The figure shows three views and two pictorial views of one solid part (mm, origin at its lowest corner). Answer the questions. A direction names the side the tool comes from. Coordinates: 2 decimals unless noted, no trailing zeros. Loops run counter-clockwise (first coordinate to the right, second up) from the corner with the lowest first, then second, coordinate; pieces in that order, holes last. Notation, with made-up numbers: M -4,55.25 L 46,55.25 A24 cw 46,71.25 Z; hole C 53,54 d1. An arc over 180 degrees is marked long. Answer as a JSON object with one key per item and string values. Group by question number.
1. For the marked faces 1, 2 and 3, determine the directions among +Z, -Z, +X, -X, +Y, -Y from which every point of the face is accessible in a straight line to the end or side of a thin tool.
2. Given pin 1 (1 mm diameter, centred on x = 58, z = 20.5, fed in from +Y); pin 2 (11 mm diameter, centred on x = 62, y = 20.5, fed in from -Z); pin 3 (1 mm diameter, centred on x = 32.5, z = 41.5, fed in from +Y) (1 decimal), each flat-ended and moving along its own axis, determine where each tip first touches the part or whether it passes through.
3. Determine the mould class of the marked faces 4, 5 and 6 for opening direction X: released by +X, released by -X, zero draft, split by the parting line, or undercut.
4. A cutting plane is placed at C-C on x = 66. Give the vertices of the cut face in (y, z) (1 decimal), and give its area (3 significant figures).
5. A cutting plane is placed at D-D on x = 20. Give the vertices of the cut face in (y, z), and give its area (3 significant figures).
6. Straight lines are drawn through the part: L1, parallel to Z at x = 61, y = 81.5; L2, parallel to Y at x = 31, z = 54; L3, parallel to Y at x = 54.5, z = 52 (1 decimal). For each, find the intervals that lie inside material, in ascending order.
7. A cutting plane is placed at A-A on y = 34. Give the vertices of the cut face in (x, z).
8. A cutting plane is placed at B-B on z = 43.5. Give the vertices of the cut face in (x, y).
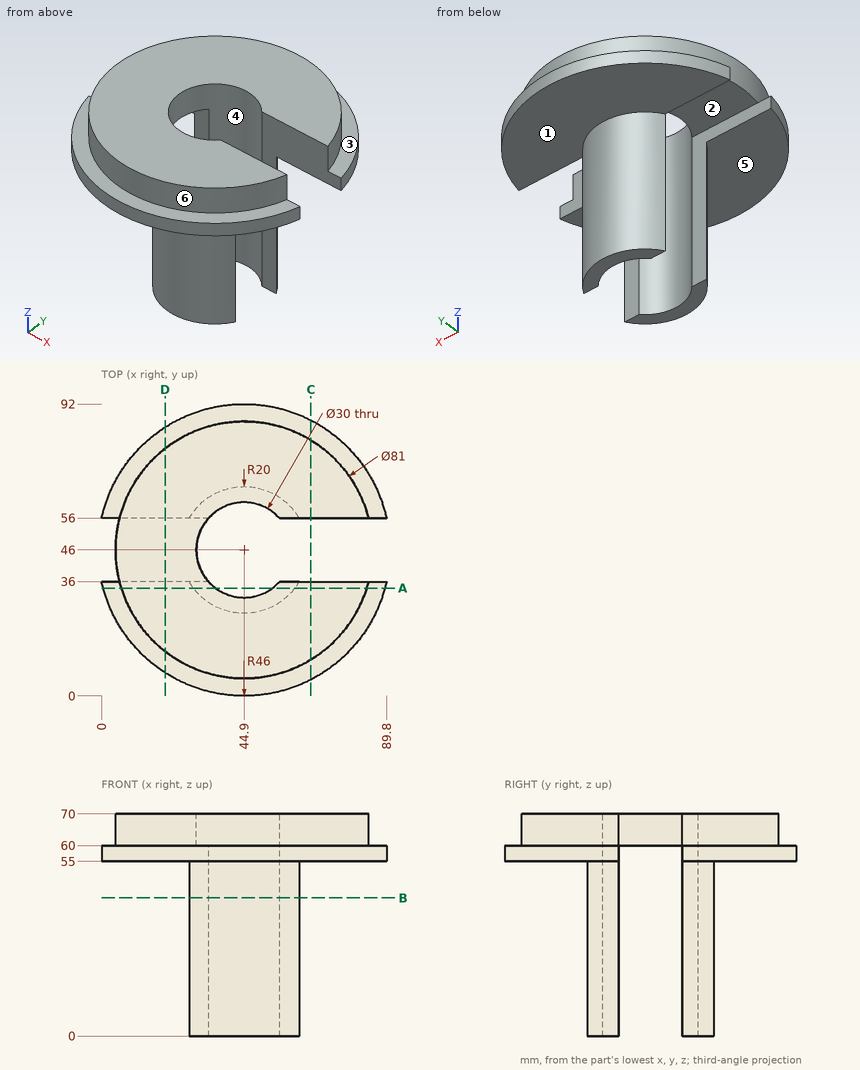
From the geometry:
{
 "1": {"face 1": "-Z, +Y", "face 2": "-Z, +X, -X", "face 3": "+Z, +Y"},
 "2": {"pin 1": "stops at y = 61.53", "pin 2": "stops at z = 55", "pin 3": "stops at y = 62.1"},
 "3": {"face 4": "undercut", "face 5": "zero draft", "face 6": "split by the parting line"},
 "4": {"outline": "M 5.1,55 L 36,55 L 36,70 L 11.4,70 L 11.4,60 L 5.1,60 Z; M 56,55 L 86.9,55 L 86.9,60 L 80.6,60 L 80.6,70 L 56,70 Z", "area": "800 mm²"},
 "5": {"outline": "M 7.32,55 L 36,55 L 36,60 L 56,60 L 56,55 L 84.68,55 L 84.68,60 L 77.94,60 L 77.94,70 L 14.06,70 L 14.06,60 L 7.32,60 Z", "area": "926 mm²"},
 "6": {"L1": "z = 55 to 70", "L2": "y = 31.62 to 36, 56 to 60.38", "L3": "y = 28.5 to 34.5, 57.5 to 63.5"},
 "7": {"outline": "M 0.49,55 L 28.9,55 L 28.9,0 L 35.9,0 L 35.9,70 L 6.22,70 L 6.22,60 L 0.49,60 Z; M 53.9,0 L 60.9,0 L 60.9,55 L 89.31,55 L 89.31,60 L 83.58,60 L 83.58,70 L 53.9,70 Z"},
 "8": {"outline": "M 27.58,36 A20 ccw 62.22,36 L 56.08,36 A15 cw 33.72,36 Z; M 27.58,56 L 33.72,56 A15 cw 56.08,56 L 62.22,56 A20 ccw Z"}
}
